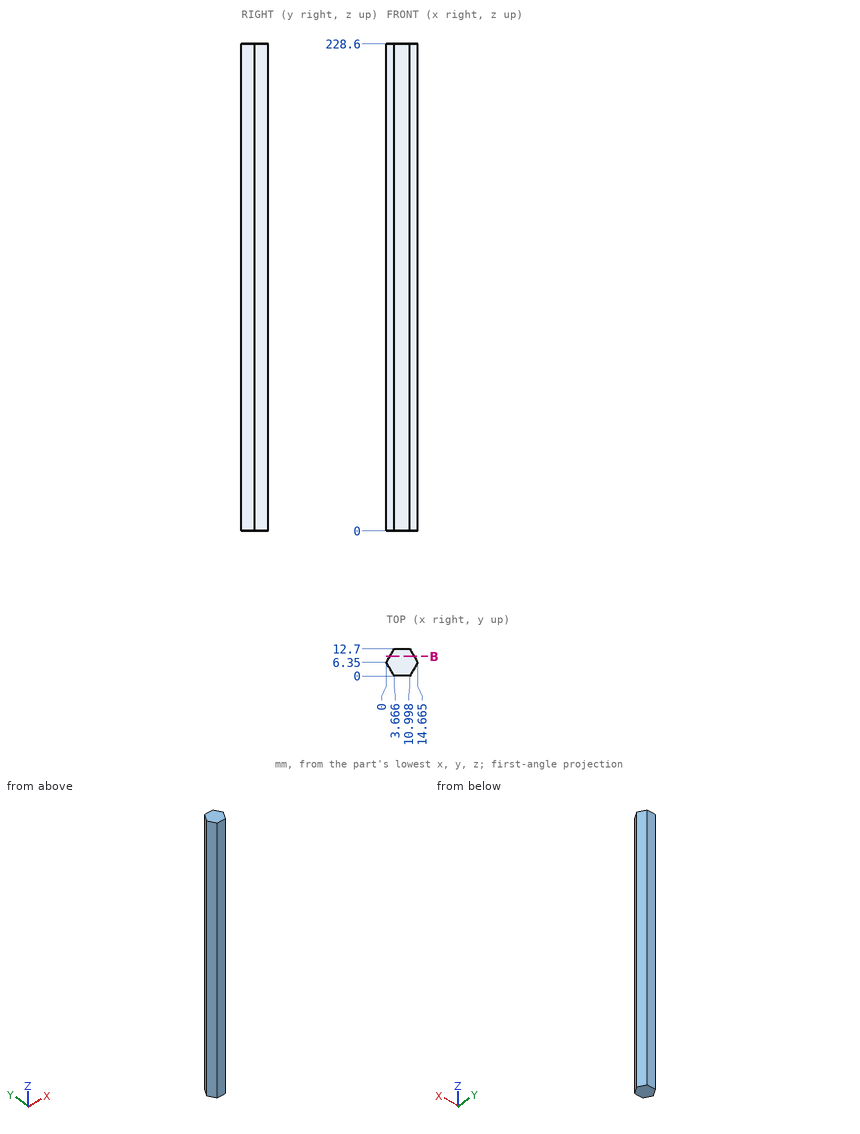
For this review, use the dimensioned drawing (mm, ordinates from the lowest corner) and the shaded views. Coordinates: 2 decimals unless noted, no trailing zeros. Loops run counter-clockwise (first coordinate to the right, second up) from the corner with the lowest first, then second, coordinate; pieces in that order, holes last. Notation, with made-up numbers: (17, 39) - (67, 39) arc R30 ccw to (67, 72) - close; hole circle Ø1 at (60.5, 68.5). An arc over 180 degrees is marked (long way). Use one line per item in the form item = value. Start each with the question number.
1) To check wall thickness, follow probe 1 along X at (y, z) = (3.75, 60) (1 decimal); probe 2 along X at (y, z) = (6.75, 155.5) (1 decimal); probe 3 along Y at (x, z) = (12.75, 13) (1 decimal). State the ranges of each line that lie inside material, in increasing order. Write a range as from..to.
2) Take a section at B-B (y = 9.25). State the section outline as (x, z) points (1 decimal), plus the area to 3 significant figures.
3) For pin 1 (3 mm diameter, centred on y = 1.5, z = 43, fed in from +X), flat-tipped, find the tip position at first contact; note if it passes through.
From the geometry:
q1.probe_1 = 1.5..13.2
q1.probe_2 = 0.2..14.4
q1.probe_3 = 3..9.7
q2.outline = (1.7, 0) - (13, 0) - (13, 228.6) - (1.7, 228.6) - close
q2.area = 2,590 mm2
q3.pin_1 = 12.73
